```python
from build123d import *

# Parameters (mm, degrees)
F0_R     = 45
F1_DEPTH = 10
F2_T     = -2.5
F3_W     = 92
F3_H     = 92
F4_DEPTH = 2
F5_R     = 2
F6_DEPTH = 6
F7_R     = 1


with BuildPart() as f1:
    # F0 (on Top) → F1 (new body)
    with BuildSketch(Plane.XY):
        Circle(F0_R)
    extrude(amount=-F1_DEPTH)

    # F2
    f2_openings = [f1.faces().sort_by_distance(p)[0] for p in [
        (0, 0, 0),
        (0, 0, -10),
    ]]
    offset(amount=F2_T, openings=f2_openings)

    # F3 (on face) → F4 (join)
    with BuildSketch(Plane.XY):
        Rectangle(F3_W, F3_H)
    extrude(amount=F4_DEPTH)

    # F5 (on face) → F6 (cut)
    with BuildSketch(Plane(origin=(0, 0, 0), x_dir=(1, 0, 0), z_dir=(0, 0, -1))):
        with Locations((-7.6630815103, 32.1338913288)):
            Circle(F5_R)
        with Locations((12.6882642508, 30.5011104792)):
            Circle(F5_R)
        with Locations((28.1931243262, 17.2179421212)):
            Circle(F5_R)
        with Locations((32.9291691581, -2.6418949108)):
            Circle(F5_R)
        with Locations((25.0873905929, -21.4926178815)):
            Circle(F5_R)
        with Locations((-25.0873905929, 21.4926178815)):
            Circle(F5_R)
        with Locations((-32.9291691581, 2.6418949108)):
            Circle(F5_R)
        with Locations((-28.1931243262, -17.2179421212)):
            Circle(F5_R)
        with Locations((-12.6882642508, -30.5011104792)):
            Circle(F5_R)
        with Locations((7.6630815103, -32.1338913288)):
            Circle(F5_R)
    extrude(amount=-F6_DEPTH, mode=Mode.SUBTRACT)

    # F7
    f7_edges = [f1.edges().sort_by_distance(p)[0] for p in [
        (-45, 0, -10),
        (-42.5, 0, -10),
    ]]
    fillet(f7_edges, radius=F7_R)


solid = f1.part
```
Source: CAD feature listing. Evaluate the final solid. Frame: model axes, mm. A direction names the side the tool comes from. Give positions to 0.01 mm unless a question says otherwise; leave off trailing zeros. Loops run counter-clockwise (first coordinate to the right, second up) from the corner with the lowest first, then second, coordinate; pieces in that order, holes last. Notation, with made-up numbers: (50.5, -21.5) -> (66.5, -21.5) arc R14 cw to (66.5, 2.5) -> close; hole circle Ø7 at (-7.5, 82.25). An arc over 180 degrees is marked (long way). Use a Markdown table: item, result. Add a question column.
(1) Pull-direction query (X, two-part tool) for faces 1 (the face through (-46, -1, 1)), 2 (the face through (23.09, 21.4, 0.99)), 3 (the face through (-45, 7, 0)); classes: +X half, -X half, draft (parallel to the pull), parting line (faces both ways), or undercut.
(2) Section query A-A (x = 0). Output: boundary loops of the cut face in (y, z).
(3) Access query for faces 4 (the face through (-1, 46, 1)), 5 (the face through (-1, 1, 0)). Directions: +Z, -Z, +X, -X, +Y, -Y. A direction counts if a zero-diameter tool reaches every point of the face in a straight line with its end or side. Return the directions, or none.
(4) First-contact query: pin 1 Ø2 at (x, z) = (33, -8.5) entering from +Y; pin 2 Ø4 at (x, y) = (9.5, 19.5) entering from -Z; pin 3 Ø5 at (x, z) = (36, -3) entering from +Y. Flat tips, straight axial feed; report the tip coordinate or a pass-through.
(5) Ray query, line 1 (Y direction, x = 0, z = -3.5); line 2 (Z direction, x = 29, y = -2.5); line 3 (Y direction, x = -25, z = -3). Return the intervals inside material, ascending.
Checked values:
| question | item | result |
|---|---|---|
| 1 | face 1 | -X half |
| 1 | face 2 | undercut |
| 1 | face 3 | draft |
| 2 | outline | (-46, 0) -> (-45, 0) -> (-45, -9) arc R1 ccw to (-44, -10) -> (-43.5, -10) arc R1 ccw to (-42.5, -9) -> (-42.5, 0) -> (42.5, 0) -> (42.5, -9) arc R1 ccw to (43.5, -10) -> (44, -10) arc R1 ccw to (45, -9) -> (45, 0) -> (46, 0) -> (46, 2) -> (-46, 2) -> close |
| 3 | face 4 | +Z, -Z, +X, -X, +Y |
| 3 | face 5 | -Z |
| 4 | pin 1 | y = 31.64 |
| 4 | pin 2 | z = 0 |
| 4 | pin 3 | y = 30.05 |
| 5 | line 1 | -45 to -42.5, 42.5 to 45 |
| 5 | line 2 | 0 to 2 |
| 5 | line 3 | -37.42 to -34.37, 34.37 to 37.42 |
